The listing builds one solid part. Answer for the finished solid, in the listing's coordinates (mm). A direction names the side the tool comes from. Coordinates: 2 decimals unless noted, no trailing zeros. Write each loop counter-clockwise with the first axis right and the second up, starting at its lowest first coordinate (ties: lowest second). Pieces come first, ordered by that corner, then holes.
from build123d import *

# Parameters (mm, degrees)
SKETCH1_W           = 31.5
SKETCH1_H           = 31.5
BOSS_EXTRUDE1_DEPTH = 110
SKETCH2_R           = 14.25
CUT_EXTRUDE1_DEPTH  = 108
BOSS_EXTRUDE2_DEPTH = 1.5
BOSS_EXTRUDE3_DEPTH = 1.5
BOSS_EXTRUDE4_DEPTH = 31.5
SKETCH10_W          = 31.5
SKETCH10_H          = 3
BOSS_EXTRUDE5_DEPTH = 55
SKETCH9_W           = 15
SKETCH9_H           = 31.5
CUT_EXTRUDE4_DEPTH  = 25
BOSS_EXTRUDE6_DEPTH = 1.5
BOSS_EXTRUDE7_DEPTH = 3
BOSS_EXTRUDE8_DEPTH = 3
BOSS_EXTRUDE9_START = 4.5
BOSS_EXTRUDE9_DEPTH = 4.5
SKETCH7_R           = 1.75
SKETCH7_R_2         = 7.5
CUT_EXTRUDE3_DEPTH  = 17.25


with BuildPart() as part:
    # Sketch1 → Boss-Extrude1 (new body)
    with BuildSketch(Plane(origin=(0, 0, 0), x_dir=(1, 0, 0), z_dir=(0, 1, 0))):
        with Locations((15.75, -15.75)):
            Rectangle(SKETCH1_W, SKETCH1_H)
    extrude(amount=BOSS_EXTRUDE1_DEPTH)

    # Sketch2 → Cut-Extrude1 (cut)
    with BuildSketch(Plane(origin=(0, 110, 0), x_dir=(1, 0, 0), z_dir=(0, 1, 0))):
        with Locations(Location((15.75, -15.75, 0), (0, 0, 270))):
            Circle(SKETCH2_R)
    extrude(amount=-CUT_EXTRUDE1_DEPTH, mode=Mode.SUBTRACT)

    # Sketch4 → Boss-Extrude2 (add)
    with BuildSketch(Plane.ZY):
        with BuildLine():
            Line((33.91386173, 122.48942639), (31.5, 110))
            Line((31.5, 110), (25.037087811, 110))
            ThreePointArc((25.037087811, 110), (15.75, 107.5), (6.462912189, 110))
            Line((6.462912189, 110), (0, 110))
            Line((0, 110), (-2.41386173, 122.48942639))
            ThreePointArc((-2.41386173, 122.48942639), (15.75, 144.5), (33.91386173, 122.48942639))
        make_face()
    extrude(amount=-BOSS_EXTRUDE2_DEPTH)

    # Sketch4<3> → Boss-Extrude3 (add)
    with BuildSketch(Plane.ZY):
        with BuildLine():
            Line((33.91386173, 122.48942639), (31.5, 110))
            Line((31.5, 110), (25.037087811, 110))
            ThreePointArc((25.037087811, 110), (15.75, 107.5), (6.462912189, 110))
            Line((6.462912189, 110), (0, 110))
            Line((0, 110), (-2.41386173, 122.48942639))
            ThreePointArc((-2.41386173, 122.48942639), (15.75, 144.5), (33.91386173, 122.48942639))
        make_face()
    extrude(amount=-BOSS_EXTRUDE3_DEPTH)

    # Sketch6 → Boss-Extrude4 (add)
    with BuildSketch(Plane.XY.offset(31.5)):
        Polygon((0, 90), (0, 110), (-4.5, 110), (-4.5, 105), align=None)
    extrude(amount=-BOSS_EXTRUDE4_DEPTH)

    # Sketch10 → Boss-Extrude5 (add)
    with BuildSketch(Plane.ZY):
        with Locations((15.75, 1.5)):
            Rectangle(SKETCH10_W, SKETCH10_H)
    extrude(amount=BOSS_EXTRUDE5_DEPTH)

    # Sketch9 → Cut-Extrude4 (cut)
    with BuildSketch(Plane(origin=(0, 110, 0), x_dir=(1, 0, 0), z_dir=(0, 1, 0))):
        with Locations((15.75, -15.75)):
            Rectangle(SKETCH9_W, SKETCH9_H)
    extrude(amount=-CUT_EXTRUDE4_DEPTH, mode=Mode.SUBTRACT)

    # Sketch14 → Boss-Extrude6 (add, symmetric)
    with BuildSketch(Plane(origin=(0, 0, 15.75), x_dir=(-1, 0, 0), z_dir=(0, 0, -1))):
        Polygon((55, 3), (0, 48), (0, 3), align=None)
    extrude(amount=BOSS_EXTRUDE6_DEPTH, both=True)

    # Sketch15 → Boss-Extrude7 (add)
    with BuildSketch(Plane.XY.offset(31.5)):
        Polygon((8.25, 110), (1.5, 110), (1.5, 122), align=None)
    extrude(amount=-BOSS_EXTRUDE7_DEPTH)

    # Sketch16 → Boss-Extrude8 (add)
    with BuildSketch(Plane(origin=(0, 0, 0), x_dir=(-1, 0, 0), z_dir=(0, 0, -1))):
        Polygon((-8.25, 110), (-1.5, 110), (-1.5, 122), align=None)
    extrude(amount=-BOSS_EXTRUDE8_DEPTH)

    # Sketch4<4> → Boss-Extrude9 (add)
    with BuildSketch(Plane.ZY.offset(BOSS_EXTRUDE9_START)):
        with BuildLine():
            Line((33.91386173, 122.48942639), (31.5, 110))
            Line((31.5, 110), (25.037087811, 110))
            ThreePointArc((25.037087811, 110), (15.75, 107.5), (6.462912189, 110))
            Line((6.462912189, 110), (0, 110))
            Line((0, 110), (-2.41386173, 122.48942639))
            ThreePointArc((-2.41386173, 122.48942639), (15.75, 144.5), (33.91386173, 122.48942639))
        make_face()
    extrude(amount=-BOSS_EXTRUDE9_DEPTH)

    # Sketch7 → Cut-Extrude3 (cut, symmetric)
    with BuildSketch(Plane(origin=(1.5, 0, 0), x_dir=(0, 0, -1), z_dir=(1, 0, 0))):
        with Locations(Location((-31.25, 126, 0), (0, 0, 270))):
            Circle(SKETCH7_R)
        with Locations(Location((-23.5, 139.423393759, 0), (0, 0, 270))):
            Circle(SKETCH7_R)
        with Locations(Location((-8, 139.423393759, 0), (0, 0, 270))):
            Circle(SKETCH7_R)
        with Locations(Location((-0.25, 126, 0), (0, 0, 270))):
            Circle(SKETCH7_R)
        with Locations(Location((-15.75, 119, 0), (0, 0, 270))):
            Circle(SKETCH7_R_2)
    extrude(amount=CUT_EXTRUDE3_DEPTH, both=True, mode=Mode.SUBTRACT)


solid = part.part
Q1. The part is cut by section C-C, the plane y = 75. Write down the section's boundary in (x, z), then the cut area to 3 significant figures.
Answers below:
outline: (0, 0) - (31.5, 0) - (31.5, 31.5) - (0, 31.5) - close; hole circle Ø28.5 at (15.75, 15.75)
area: 354 mm2
Q2. Given pin 1 (2 mm diameter, centred on x = 3.5, z = 25, fed in from +Y); pin 2 (10 mm diameter, centred on y = 56, z = 29.5, fed in from -X); pin 3 (5 mm diameter, centred on x = 15.5, y = 49, fed in from -Z); pin 4 (2 mm diameter, centred on x = 20, z = 29.5, fed in from -Y), each flat-ended and moving along its own axis, determine where each tip first touches the part or whether it passes through.
Answers below:
pin 1: stops at y = 110
pin 2: stops at x = 0
pin 3: stops at z = 0
pin 4: stops at y = 0
Q3. Find the intervals of material crossed by probe 1 along X at (y, z) = (54, 15.75); probe 2 along Z at (x, y) = (12, 58); probe 3 along X at (y, z) = (108, 2), in increasing order.
Answers below:
probe 1: x = 0 to 1.5, 30 to 31.5
probe 2: z = 0 to 2, 29.5 to 31.5
probe 3: x = -4.5 to 8.25, 23.25 to 31.5
Q4. The part is cut by section D-D, the plane x = -35.5. Write down the section's boundary in (y, z).
Answers below:
outline: (0, 0) - (3, 0) - (3, 14.25) - (18.95, 14.25) - (18.95, 17.25) - (3, 17.25) - (3, 31.5) - (0, 31.5) - close
Q5. Which of the six approach directions +Z, -Z, +X, -X, +Y, -Y give full straight-line access (tool end or side, diameter ignored) to faces 1 (the face through (-4.5, 129, 16)), 2 (the face through (16.377, 56.756, 1.514)), 3 (the face through (1.5, 127, 16)), 4 (the face through (23.25, 98, 30))?
Answers below:
face 1: +Z, -Z, -X, +Y
face 2: +Y
face 3: +X, +Y
face 4: +Z, -Z, +Y
Q6. Determine the mould class of faces 5 (the face through (23.25, 98, 2)), 6 (the face through (0, 47, 12)), 7 (the face through (-1.5, 116.2, -1.2)) for opening direction Y: released by +Y, released by -Y, zero draft, split by the parting line, or undercut.
Answers below:
face 5: zero draft
face 6: undercut
face 7: released by -Y
Q7. The part is cut by section A-A, the plane x = 15.75. Write down the section's boundary in (y, z), then the cut area to 3 significant figures.
Answers below:
outline: (0, 0) - (85, 0) - (85, 1.5) - (2, 1.5) - (2, 30) - (85, 30) - (85, 31.5) - (0, 31.5) - close
area: 312 mm2
Q8. The part is cut by section B-B, the plane y = 119. Write down the section's boundary in (x, z).
Answers below:
outline: (-4.5, -1.74) - (1.5, -1.74) - (1.5, 0) - (3.19, 0) - (3.19, 3) - (1.5, 3) - (1.5, 8.25) - (-4.5, 8.25) - close; (-4.5, 23.25) - (1.5, 23.25) - (1.5, 28.5) - (3.19, 28.5) - (3.19, 31.5) - (1.5, 31.5) - (1.5, 33.24) - (-4.5, 33.24) - close
